Read the model definition and answer for the solid it produces. Units are mm, in the model's axes. A direction names the side the tool comes from. Coordinates: 2 decimals unless noted, no trailing zeros. Write each loop counter-clockwise with the first axis right and the second up, starting at its lowest first coordinate (ties: lowest second). Pieces come first, ordered by that corner, then holes. Notation, with made-up numbers: (-28, 25.25) - (14, 25.25) arc R18 ccw to (14, 41.25) - close; hole circle Ø8 at (21, 2). An arc over 180 degrees is marked (long way). Return JSON: item names as keys, results as strings.
```python
from build123d import *

# Parameters (mm, degrees)
SKETCH1_R           = 1.445
BOSS_EXTRUDE1_DEPTH = 1.5
SKETCH2_W           = 43
SKETCH2_H           = 17.6
BOSS_EXTRUDE2_DEPTH = 7
SKETCH3_W           = 9.25
SKETCH3_H           = 7.5
BOSS_EXTRUDE3_DEPTH = 4.35
SKETCH4_W           = 3.39
SKETCH4_H           = 5.8
BOSS_EXTRUDE4_DEPTH = 8.42
SKETCH5_W           = 14
SKETCH5_H           = 15
BOSS_EXTRUDE5_DEPTH = 8
SKETCH6_W           = 12.25
SKETCH6_H           = 16.5
BOSS_EXTRUDE6_DEPTH = 12


with BuildPart() as part:
    # Sketch1 → Boss-Extrude1 (new body)
    with BuildSketch(Plane(origin=(0, 0, 0), x_dir=(1, 0, 0), z_dir=(0, 1, 0))):
        with BuildLine():
            Line((-35.7, 28.5), (35.7, 28.5))
            ThreePointArc((35.7, 28.5), (42.771067812, 25.571067812), (45.7, 18.5))
            Line((45.7, 18.5), (45.7, -18.5))
            ThreePointArc((45.7, -18.5), (42.771067812, -25.571067812), (35.7, -28.5))
            Line((35.7, -28.5), (-35.7, -28.5))
            ThreePointArc((-35.7, -28.5), (-42.771067812, -25.571067812), (-45.7, -18.5))
            Line((-45.7, -18.5), (-45.7, 18.5))
            ThreePointArc((-45.7, 18.5), (-42.771067812, 25.571067812), (-35.7, 28.5))
        make_face()
        with Locations(Location((-38.05, 20.85, 0), (0, 0, 270))):
            Circle(SKETCH1_R, mode=Mode.SUBTRACT)
        with Locations(Location((-38.05, -20.85, 0), (0, 0, 270))):
            Circle(SKETCH1_R, mode=Mode.SUBTRACT)
        with Locations(Location((38.05, 20.85, 0), (0, 0, 270))):
            Circle(SKETCH1_R, mode=Mode.SUBTRACT)
        with Locations(Location((38.05, -20.85, 0), (0, 0, 270))):
            Circle(SKETCH1_R, mode=Mode.SUBTRACT)
    extrude(amount=BOSS_EXTRUDE1_DEPTH)

    # Sketch2 → Boss-Extrude2 (add)
    with BuildSketch(Plane(origin=(0, 1.5, 0), x_dir=(1, 0, 0), z_dir=(0, 1, 0))):
        with Locations((-21.05, 1.3)):
            Rectangle(SKETCH2_W, SKETCH2_H)
    extrude(amount=BOSS_EXTRUDE2_DEPTH)

    # Sketch3 → Boss-Extrude3 (add)
    with BuildSketch(Plane(origin=(0, 8.5, 0), x_dir=(1, 0, 0), z_dir=(0, 1, 0))):
        with Locations((-40.125, 1.3)):
            Rectangle(SKETCH3_W, SKETCH3_H)
    extrude(amount=BOSS_EXTRUDE3_DEPTH)

    # Sketch4 → Boss-Extrude4 (add)
    with BuildSketch(Plane(origin=(0, 8.5, 0), x_dir=(1, 0, 0), z_dir=(0, 1, 0))):
        with Locations((-2.245, 1.3)):
            Rectangle(SKETCH4_W, SKETCH4_H)
    extrude(amount=BOSS_EXTRUDE4_DEPTH)

    # Sketch5 → Boss-Extrude5 (add)
    with BuildSketch(Plane(origin=(0, 1.5, 0), x_dir=(1, 0, 0), z_dir=(0, 1, 0))):
        with Locations((45.7, 2.3)):
            Rectangle(SKETCH5_W, SKETCH5_H)
    extrude(amount=BOSS_EXTRUDE5_DEPTH)

    # Sketch6 → Boss-Extrude6 (add)
    with BuildSketch(Plane(origin=(0, 1.5, 0), x_dir=(1, 0, 0), z_dir=(0, 1, 0))):
        with Locations((25.637075285, -27.25)):
            Rectangle(SKETCH6_W, SKETCH6_H)
    extrude(amount=BOSS_EXTRUDE6_DEPTH)


solid = part.part
```
(1) Flat-ended cylindrical pins translate along their axes: P1, Ø2, axis at x = 25, z = 32.5, coming from the -Y side; P2, Ø13.5, axis at x = 28, z = 29, coming from the +Y side; P3, Ø6, axis at x = -40, z = -2, coming from the +Y side; P4, Ø1, axis at x = -34.5, y = 14, coming from the -Z side. Find the tip coordinate at first contact, or state that the pin passes through.
Answer:
{"P1": "y = 1.5", "P2": "y = 13.5", "P3": "y = 12.85", "P4": "through"}
(2) Determine the mould class of faces 1 (the face through (38.7, 5, -2)), 2 (the face through (-42.69, 0.74, 25.65)), 3 (the face through (-36.832, 0.74, -20.073)), 4 (the face through (-40, 11, 2.45)) for opening direction X: +X half, -X half, draft (parallel to the pull), parting line (faces both ways), or undercut.
Answer:
{"face 1": "undercut", "face 2": "-X half", "face 3": "undercut", "face 4": "draft"}
(3) A cutting plane is placed at B-B (y = 3.5). Determine the outline of the cut face in (x, z).
Answer:
{"outline": "(-42.55, -10.1) - (0.45, -10.1) - (0.45, 7.5) - (-42.55, 7.5) - close; (19.51, 19) - (31.76, 19) - (31.76, 35.5) - (19.51, 35.5) - close; (38.7, -9.8) - (52.7, -9.8) - (52.7, 5.2) - (38.7, 5.2) - close"}
(4) A cutting plane is placed at C-C (z = -20.85). Determine the outline of the cut face in (x, y) (3 decimals).
Answer:
{"outline": "(-45.42, 0) - (-39.495, 0) - (-39.495, 1.5) - (-45.42, 1.5) - close; (-36.605, 0) - (36.605, 0) - (36.605, 1.5) - (-36.605, 1.5) - close; (39.495, 0) - (45.42, 0) - (45.42, 1.5) - (39.495, 1.5) - close"}
(5) Straight lines are drawn through the part: line 1 (X direction, y = 1.1, z = 20.85) (3 decimals); line 2 (Z direction, x = -6, y = 1); line 3 (X direction, y = 2, z = -10). For each, find the intervals that lie inside material, in ascending order. Write a range as from..to.
Answer:
{"line 1": "-45.42..-39.495, -36.605..36.605, 39.495..45.42", "line 2": "-28.5..28.5", "line 3": "-42.55..0.45"}
(6) A cutting plane is placed at A-A (x = -7). Determine the outline of the cut face in (y, z).
Answer:
{"outline": "(0, -28.5) - (1.5, -28.5) - (1.5, -10.1) - (8.5, -10.1) - (8.5, 7.5) - (1.5, 7.5) - (1.5, 28.5) - (0, 28.5) - close"}
(7) Which of the six approach directions +Z, -Z, +X, -X, +Y, -Y give full straight-line access (tool end or side, diameter ignored) to faces 5 (the face through (-21, 5, 7.5)), 6 (the face through (31.762, 7, 27)), 7 (the face through (26, 1.5, 32))?
Answer:
{"face 5": "+Z, +X, -X, +Y", "face 6": "+Z, -Z, +X, +Y", "face 7": "+Z, +X, -X, -Y"}
(8) A cutting plane is placed at D-D (x = -38.05). Determine the outline of the cut face in (y, z) (3 decimals).
Answer:
{"outline": "(0, -28.22) - (1.5, -28.22) - (1.5, -22.295) - (0, -22.295) - close; (0, -19.405) - (1.5, -19.405) - (1.5, -10.1) - (8.5, -10.1) - (8.5, -5.05) - (12.85, -5.05) - (12.85, 2.45) - (8.5, 2.45) - (8.5, 7.5) - (1.5, 7.5) - (1.5, 19.405) - (0, 19.405) - close; (0, 22.295) - (1.5, 22.295) - (1.5, 28.22) - (0, 28.22) - close"}
